The listing builds one solid part. Answer for the finished solid, in the listing's coordinates (mm). Round coordinates to 2 decimals unless told otherwise and drop trailing zeros. Write each loop counter-clockwise with the first axis right and the second up, starting at its lowest first coordinate (ties: lowest second). Pieces come first, ordered by that corner, then holes.
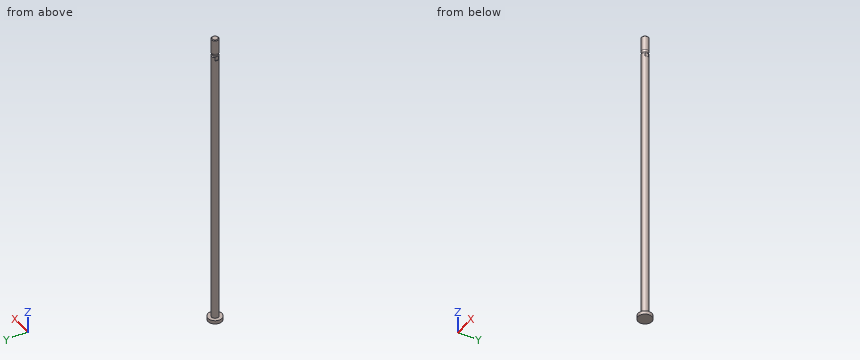
Autodesk Inventor part; units mm, degrees
ref_plane "FDT_KSAUFSATZ_XY" through (0, 0, 11.2) normal (0, 0, 1) x (-1, 0, 0)
ref_plane "FDT_KSAUFSATZ_YZ" through (0, 0, 11.2) normal (-1, 0, 0) x (0, -1, 0)
ref_plane "FDT_KSAUFSATZ_ZX" through (0, 0, 11.2) normal (0, -1, 0) x (0, 0, 1)
sketch "Sketch_2" plane through (0, 0, 0) normal (1, 0, 0) x (0, 1, 0)
  line L0 (0, -240.3) -> (0, 5)
  line L1 (0, 5) -> (3, 5)
  line L2 (3, 5) -> (3, -237.3)
  line L3 (3, -237.3) -> (6, -237.3)
  line L4 (6, -237.3) -> (6, -240.3)
  line L5 (6, -240.3) -> (0, -240.3)
  line L6 (0, -240.3) -> (0, 5)
revolve "Revolution1" add sketch "Sketch_2" angle 360 about axis through (0, 0, -240.3) along (0, 0, -1)
sketch "Sketch_6" plane through (0, 0, 0) normal (1, 0, 0) x (0, 1, 0)
  line L0 (0, 4) -> (0, 21)
  line L1 (0, 21) -> (2.3865, 21)
  line L2 (2.3865, 21) -> (3, 20.3865)
  line L3 (3, 20.3865) -> (3, 8.1485)
  line L4 (3, 8.1485) -> (2.4362, 6.5994)
  arc A0 (2.4362, 6.5994) -> (2.4, 6.3942) centre (3, 6.3942) ccw
  line L5 (2.4, 6.3942) -> (2.4, 5.6)
  arc A1 (2.4, 5.6) -> (3, 5) centre (3, 5.6) ccw
  line L6 (3, 5) -> (3, 4)
  line L7 (3, 4) -> (0, 4)
  line L8 (0, 4) -> (0, 21)
revolve "Revolution2" add sketch "Sketch_6" angle 360 about axis through (0, 0, 4) along (0, 0, -1)
thread "Thread1"
sketch "Sketch_7" plane through (0, 0, 2) normal (0, 0, 1) x (1, 0, 0)
  line L0 (-5, 10) -> (-5, -5)
  line L1 (-5, -5) -> (-2.5, -5)
  line L2 (-2.5, -5) -> (-2.5, 5)
  line L3 (-2.5, 5) -> (2.5, 5)
  line L4 (2.5, 5) -> (2.5, -5)
  line L5 (2.5, -5) -> (5, -5)
  line L6 (5, -5) -> (5, 10)
  line L7 (5, 10) -> (-5, 10)
extrude "Extrusion1" cut sketch "Sketch_7" along normal blind 4
ref_plane "FDT_KSAUFSATZ_XY" through (0, 0, 11.2) normal (0, 0, 1) x (-1, 0, 0)
ref_plane "FDT_KSAUFSATZ_YZ" through (0, 0, 11.2) normal (-1, 0, 0) x (0, -1, 0)
ref_plane "FDT_KSAUFSATZ_ZX" through (0, 0, 11.2) normal (0, -1, 0) x (0, 0, 1)
ref_plane "FDT_NUT_XY" through (0, 0, 11.2) normal (0, 0, 1) x (-1, 0, 0)
ref_plane "FDT_NUT_YZ" through (0, 0, 11.2) normal (-1, 0, 0) x (0, -1, 0)
ref_plane "FDT_NUT_ZX" through (0, 0, 11.2) normal (0, -1, 0) x (0, 0, 1)
ref_plane "KS_XY" through (0, 0, 0) normal (0, 0, -1) x (1, 0, 0)
ref_plane "KS_YZ" through (0, 0, 0) normal (1, 0, 0) x (0, -1, 0)
ref_plane "KS_ZX" through (0, 0, 0) normal (0, -1, 0) x (0, 0, -1)
ref_plane "NUT1_XY" through (0, 0, 16) normal (0, 0, 1) x (1, 0, 0)
ref_plane "NUT1_YZ" through (0, 0, 16) normal (1, 0, 0) x (0, 1, 0)
ref_plane "NUT1_ZX" through (0, 0, 16) normal (0, 1, 0) x (0, 0, 1)
properties part number "19197 DSNU-12-200-P---(A---00--0-KS)"
1. Section A-A on z = -79 is taken. Determine the outline of the cut face in (x, y), plus the area to 3 significant figures.
Geometry says:
outline: circle Ø6 at (0, 0)
area: 28.3 mm2
2. Given pin 1 (2.5 mm diameter, centred on y = 0, z = 3.5, fed in from +X); pin 2 (2.5 mm diameter, centred on y = 0, z = 4, fed in from -X); pin 3 (0.6 mm diameter, centred on x = 3, y = 0.5, fed in from +Z); pin 4 (0.6 mm diameter, centred on x = -2.5, y = 0.5, fed in from +Z), each flat-ended and moving along its own axis, determine where each tip first touches the part or whether it passes through.
Geometry says:
pin 1: stops at x = 2.5
pin 2: stops at x = -2.5
pin 3: stops at z = 20.65
pin 4: stops at z = 21
3. Straight lines are drawn through the part: line 1 along Z through (x, y) = (-4.75, -3); line 2 along X through (y, z) = (0.5, -196); line 3 along X through (y, z) = (-1.5, -95). For each, find the intervals that lie inside material, in ascending order.
Geometry says:
line 1: z = -240.3 to -237.3
line 2: x = -2.96 to 2.96
line 3: x = -2.6 to 2.6
